Check sheet for the modelled part. Datum: model origin and axes. Units: mm. Face numbers are marked on the shaded views. A direction names the side the tool comes from. Round coordinates to 2 decimals unless told otherwise and drop trailing zeros. Loops run counter-clockwise (first coordinate to the right, second up) from the corner with the lowest first, then second, coordinate; pieces in that order, holes last. Notation, with made-up numbers: M -19,-10.5 L -9,-10.5 A14 cw -9,12.5 Z; hole C -2.5,74.25 d3. An arc over 180 degrees is marked long. Write item = value, one per line. Start each with the question number.
(1) Set-up check for the marked faces 1 and 2: record each of +Z, -Z, +X, -X, +Y, -Y from which the full face is reachable in a straight line by a thin tool's end or side.
(2) Cross-section at A-A on x = 12.7. Record the boundary of the cut face in (y, z) (3 decimals), plus the area to 3 significant figures.
(3) Cross-section at D-D on z = 7.5. Record the boundary of the cut face in (x, y) (3 decimals).
(4) Cross-section at B-B on z = 38.1. Record the boundary of the cut face in (x, y) (3 decimals), plus the area to 3 significant figures.
(5) Cross-section at C-C on y = 65. Record the boundary of the cut face in (x, z) (3 decimals), plus the area to 4 significant figures.
(6) Scan lines: L1, parallel to Y at x = 12.7, z = 2.25 (3 decimals); L2, parallel to X at y = 44.45, z = 2.05 (3 decimals); L3, parallel to Y at x = 2.4, z = 38.1 (3 decimals). Record each from-to range of solid material in increasing order. Write a range as from..to.
(7) Go/stop test with flat-tipped pins: P1, Ø5.5, axis at y = 120.65, z = 12.7, coming from the -X side; P2, Ø7.5, axis at x = 38.1, y = 44.45, coming from the +Z side (3 decimals); P3, Ø12, axis at y = 101, z = 20, coming from the +X side (3 decimals); P4, Ø1, axis at x = 16, z = 2, coming from the +Y side. Record where each tip stops, or that it passes through.
Autodesk Inventor part; units mm, degrees
ref_plane "YZ Plane" through (0, 0, 0) normal (1, 0, 0) x (0, 1, 0)
ref_plane "XZ Plane" through (0, 0, 0) normal (0, 1, 0) x (-1, 0, 0)
ref_plane "XY Plane" through (0, 0, 0) normal (0, 0, 1) x (1, 0, 0)
sketch "Sketch1" plane through (0, 0, 0) normal (0, 1, 0) x (-1, 0, 0)
  line L0 (0, 0) -> (-3.175, 0)
  line L1 (-3.175, 0) -> (-3.175, 50.8)
  line L2 (-3.175, 50.8) -> (0, 50.8)
  line L3 (0, 50.8) -> (0, 0)
  line L4 (0, 0) -> (-50.8, 0)
  line L5 (-50.8, 0) -> (-50.8, 3.175)
  line L6 (-50.8, 3.175) -> (0, 3.175)
  line L7 (0, 3.175) -> (0, 0)
  dimension "d0" = 3.175
  dimension "d1" = 50.8
  dimension "d2" = 50.8
  dimension "d3" = 3.175
extrude "Extrusion1" add sketch "Sketch1" along normal blind 133.35
sketch "Sketch2" plane through (0, 0, 0) normal (-1, 0, 0) x (0, 0, 1)
  line L0 (0, 0) -> (50.8, 0)
  line L1 (50.8, 0) -> (50.8, 133.35)
  line L2 (0, 133.35) -> (50.8, 133.35)
  line L3 (0, 0) -> (0, 133.35)
  point P0 (12.7, 120.65)
  point P1 (38.1, 120.65)
  point P2 (38.1, 95.25)
  point P3 (12.7, 95.25)
  dimension "d6" = 12.7
  dimension "d7" = 12.7
  dimension "d8" = 12.7
  dimension "d9" = 12.7
  dimension "d10" = 12.7
  dimension "d11" = 38.1
  dimension "d12" = 12.7
  dimension "d13" = 38.1
hole "Hole1" at (0, 120.65, 12.7) at (0, 120.65, 38.1) at (0, 95.25, 38.1) at (0, 95.25, 12.7) direction (1, 0, 0) diameter 6.35 end through all
sketch "Sketch3" plane through (50.8, 0, 0) normal (0, 0, -1) x (-1, 0, 0)
  line L0 (0, 0) -> (50.8, 0)
  line L1 (50.8, 0) -> (50.8, 133.35)
  line L2 (0, 133.35) -> (50.8, 133.35)
  line L3 (0, 0) -> (0, 133.35)
  point P0 (12.7, 69.85)
  point P1 (38.1, 69.85)
  point P2 (38.1, 44.45)
  point P3 (12.7, 44.45)
  dimension "d21" = 12.7
  dimension "d22" = 12.7
  dimension "d23" = 63.5
  dimension "d24" = 63.5
  dimension "d34" = 12.7
  dimension "d35" = 88.9
  dimension "d36" = 88.9
  dimension "d37" = 12.7
sketch "Sketch4" plane through (0, 133.35, 0) normal (0, 1, 0) x (1, 0, 0)
  line L0 (0, 0) -> (0, -50.8)
  line L1 (0, -50.8) -> (3.175, -50.8)
  line L2 (3.175, -50.8) -> (3.175, -3.175)
  line L3 (3.175, -3.175) -> (50.8, -3.175)
  line L4 (50.8, -3.175) -> (50.8, 0)
  line L5 (50.8, 0) -> (0, 0)
  line L6 (50.8, 0) -> (3.175, 0)
  line L7 (3.175, 0) -> (3.175, -3.175)
  line L8 (3.175, -3.175) -> (50.8, -3.175)
  line L9 (50.8, -3.175) -> (50.8, 0)
extrude "Extrusion2" cut sketch "Sketch4" against normal blind 50.8 contours L5 L4 L3 L7
hole "Hole3" at (38.1, 69.85, 0) at (12.7, 69.85, 0) at (12.7, 44.45, 0) at (38.1, 44.45, 0) direction (0, 0, 1) diameter 6.35 end through all
properties part number "2x2 angle vertical left"
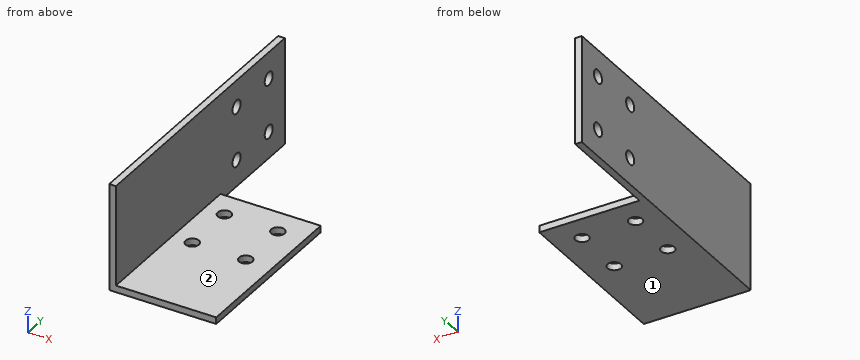
Result:
q1.face_1 = -Z, +X, -X, +Y, -Y
q1.face_2 = +Z, +X, +Y, -Y
q2.outline = M 0,0 L 41.275,0 L 41.275,3.175 L 0,3.175 Z; M 47.625,0 L 66.675,0 L 66.675,3.175 L 47.625,3.175 Z; M 73.025,0 L 82.55,0 L 82.55,3.175 L 73.025,3.175 Z
q2.area = 222 mm^2
q3.outline = M 0,0 L 3.175,0 L 3.175,133.35 L 0,133.35 Z
q4.outline = M 0,0 L 3.175,0 L 3.175,92.075 L 0,92.075 Z; M 0,98.425 L 3.175,98.425 L 3.175,117.475 L 0,117.475 Z; M 0,123.825 L 3.175,123.825 L 3.175,133.35 L 0,133.35 Z
q4.area = 383 mm^2
q5.outline = M 0,0 L 50.8,0 L 50.8,3.175 L 3.175,3.175 L 3.175,50.8 L 0,50.8 Z
q5.area = 312.5 mm^2
q6.L1 = 0..41.275, 47.625..66.675, 73.025..82.55
q6.L2 = 0..9.525, 15.875..34.925, 41.275..50.8
q6.L3 = 0..92.075, 98.425..117.475, 123.825..133.35
q7.P1 = through
q7.P2 = 3.175
q7.P3 = 3.175
q7.P4 = 82.55
